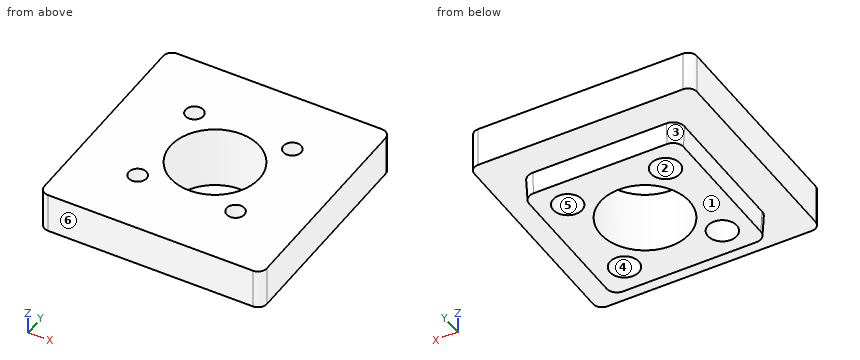
Autodesk Inventor part; units mm, degrees
ref_plane "YZ Plane" through (0, 0, 0) normal (1, 0, 0) x (0, 1, 0)
ref_plane "XZ Plane" through (0, 0, 0) normal (0, 1, 0) x (-1, 0, 0)
ref_plane "XY Plane" through (0, 0, 0) normal (0, 0, 1) x (1, 0, 0)
ref_plane "Arbeitsebene15" through (-38.58009, 58.540516, -23.010083) normal (0, 0, 1) x (1, 0, 0)
sketch "Skizze38" plane through (-38.58009, 58.540516, -23.010083) normal (0, 0, 1) x (1, 0, 0)
  circle A0 centre (27, 33.3) radius 3
  circle A1 centre (-8.3, 27) radius 3
  circle A2 centre (-2, -8.3) radius 3
  circle A3 centre (33.3, -2) radius 3
  circle A4 centre (27, -8.3) radius 3
  circle A5 centre (-8.3, -2) radius 3
  circle A6 centre (-2, 33.3) radius 3
  circle A7 centre (33.3, 27) radius 3
  line L0 (27.5, 29.5) -> (-2.5, 29.5)
  arc A8 (29.5, 27.5) -> (27.5, 29.5) centre (27.5, 27.5) ccw
  line L1 (29.5, 27.5) -> (29.5, -2.5)
  arc A9 (27.5, -4.5) -> (29.5, -2.5) centre (27.5, -2.5) ccw
  line L2 (-2.5, -4.5) -> (27.5, -4.5)
  arc A10 (-4.5, -2.5) -> (-2.5, -4.5) centre (-2.5, -2.5) ccw
  line L3 (-4.5, -2.5) -> (-4.5, 27.5)
  arc A11 (-2.5, 29.5) -> (-4.5, 27.5) centre (-2.5, 27.5) ccw
  circle A12 centre (33.5, 33.5) radius 2.5
  circle A13 centre (-8.5, -8.5) radius 2.5
  circle A14 centre (33.5, -8.5) radius 2.5
  circle A15 centre (-8.5, 33.5) radius 2.5
  line L4 (-11.75, -10.5) -> (-11.75, 8.25)
  arc A16 (-11.75, -10.5) -> (-10.5, -11.75) centre (-10.5, -10.5) ccw
  line L5 (8.25, -11.75) -> (-10.5, -11.75)
  line L6 (8.25, -13.877389) -> (8.25, -11.75)
  arc A17 (7.405556, -14.865216) -> (8.25, -13.877389) centre (7.25, -13.877389) ccw
  arc A18 (7.405556, -14.865216) -> (7.6, -17.35) centre (7.6, -16.1) ccw
  line L7 (17.4, -17.35) -> (7.6, -17.35)
  arc A19 (17.4, -17.35) -> (17.594444, -14.865216) centre (17.4, -16.1) ccw
  arc A20 (16.75, -13.877389) -> (17.594444, -14.865216) centre (17.75, -13.877389) ccw
  line L8 (16.75, -11.75) -> (16.75, -13.877389)
  line L9 (35.5, -11.75) -> (16.75, -11.75)
  arc A21 (35.5, -11.75) -> (36.75, -10.5) centre (35.5, -10.5) ccw
  line L10 (36.75, 6.487451) -> (36.75, -10.5)
  arc A22 (36.75, 6.487451) -> (36.55605, 6.521706) centre (36.65, 6.487451) ccw
  arc A23 (31.3, 7.45) -> (36.55605, 6.521706) centre (34.01, 7.45) ccw
  line L11 (31.3, 17.55) -> (31.3, 7.45)
  arc A24 (36.55605, 18.478294) -> (31.3, 17.55) centre (34.01, 17.55) ccw
  arc A25 (36.55605, 18.478294) -> (36.75, 18.512549) centre (36.65, 18.512549) ccw
  line L12 (36.75, 35.5) -> (36.75, 18.512549)
  arc A26 (36.75, 35.5) -> (35.5, 36.75) centre (35.5, 35.5) ccw
  line L13 (18.512549, 36.75) -> (35.5, 36.75)
  arc A27 (18.512549, 36.75) -> (18.478294, 36.55605) centre (18.512549, 36.65) ccw
  arc A28 (17.55, 31.3) -> (18.478294, 36.55605) centre (17.55, 34.01) ccw
  line L14 (7.45, 31.3) -> (17.55, 31.3)
  arc A29 (6.521706, 36.55605) -> (7.45, 31.3) centre (7.45, 34.01) ccw
  arc A30 (6.521706, 36.55605) -> (6.487451, 36.75) centre (6.487451, 36.65) ccw
  line L15 (-10.5, 36.75) -> (6.487451, 36.75)
  arc A31 (-10.5, 36.75) -> (-11.75, 35.5) centre (-10.5, 35.5) ccw
  line L16 (-11.75, 16.75) -> (-11.75, 35.5)
  line L17 (-13.877389, 16.75) -> (-11.75, 16.75)
  arc A32 (-14.865216, 17.594444) -> (-13.877389, 16.75) centre (-13.877389, 17.75) ccw
  arc A33 (-14.865216, 17.594444) -> (-17.35, 17.4) centre (-16.1, 17.4) ccw
  line L18 (-17.35, 7.6) -> (-17.35, 17.4)
  arc A34 (-17.35, 7.6) -> (-14.865216, 7.405556) centre (-16.1, 7.6) ccw
  arc A35 (-13.877389, 8.25) -> (-14.865216, 7.405556) centre (-13.877389, 7.25) ccw
  line L19 (-11.75, 8.25) -> (-13.877389, 8.25)
  line L20 (-2.5, 30.1) -> (27.5, 30.1)
  arc A36 (30.1, 27.5) -> (27.5, 30.1) centre (27.5, 27.5) ccw
  line L21 (30.1, 27.5) -> (30.1, -2.5)
  arc A37 (27.5, -5.1) -> (30.1, -2.5) centre (27.5, -2.5) ccw
  line L22 (27.5, -5.1) -> (-2.5, -5.1)
  arc A38 (-5.1, -2.5) -> (-2.5, -5.1) centre (-2.5, -2.5) ccw
  line L23 (-5.1, -2.5) -> (-5.1, 27.5)
  arc A39 (-2.5, 30.1) -> (-5.1, 27.5) centre (-2.5, 27.5) ccw
  point P0 (38.58009, -58.540516)
  dimension "d425" = 0.6
sketch "Skizze38 outline for Extrusion20" plane through (-38.58009, 58.540516, -23.010083) normal (0, 0, 1) x (1, 0, 0)
  arc A0 (-5.1, -2.5) -> (-2.5, -5.1) centre (-2.5, -2.5) ccw
  line L0 (-5.1, 27.5) -> (-5.1, -2.5)
  arc A1 (-2.5, 30.1) -> (-5.1, 27.5) centre (-2.5, 27.5) ccw
  line L1 (27.5, 30.1) -> (-2.5, 30.1)
  arc A2 (30.1, 27.5) -> (27.5, 30.1) centre (27.5, 27.5) ccw
  line L2 (30.1, -2.5) -> (30.1, 27.5)
  arc A3 (27.5, -5.1) -> (30.1, -2.5) centre (27.5, -2.5) ccw
  line L3 (-2.5, -5.1) -> (27.5, -5.1)
extrude "Extrusion20" add sketch "Skizze38 outline for Extrusion20" against normal blind 5 draft -3
sketch "Skizze39" plane through (-38.58009, 58.540516, -23.010083) normal (0, 0, 1) x (1, 0, 0)
  line L0 (-2.5, -5.1) -> (27.5, -5.1)
  arc A0 (27.5, -5.1) -> (30.1, -2.5) centre (27.5, -2.5) ccw
  line L1 (30.1, -2.5) -> (30.1, 27.5)
  arc A1 (30.1, 27.5) -> (27.5, 30.1) centre (27.5, 27.5) ccw
  line L2 (27.5, 30.1) -> (-2.5, 30.1)
  arc A2 (-2.5, 30.1) -> (-5.1, 27.5) centre (-2.5, 27.5) ccw
  line L3 (-5.1, 27.5) -> (-5.1, -2.5)
  arc A3 (-5.1, -2.5) -> (-2.5, -5.1) centre (-2.5, -2.5) ccw
  line L4 (17.5, -12.5) -> (35.5, -12.5)
  line L5 (-10.5, 37.5) -> (35.5, 37.5)
  line L6 (37.5, 35.5) -> (37.5, -10.5)
  line L7 (35.5, -12.5) -> (-10.5, -12.5)
  line L8 (-12.5, -10.5) -> (-12.5, 35.5)
  line L9 (-12.5, 37.5) -> (37.5, -12.5) construction
  line L10 (37.5, 37.5) -> (-12.5, -12.5) construction
  arc A4 (37.5, 35.5) -> (35.5, 37.5) centre (35.5, 35.5) ccw
  arc A5 (37.5, 35.5) -> (35.5, 37.5) centre (35.5, 35.5) ccw
  arc A6 (-10.5, 37.5) -> (-12.5, 35.5) centre (-10.5, 35.5) ccw
  arc A7 (-12.5, -10.5) -> (-10.5, -12.5) centre (-10.5, -10.5) ccw
  arc A8 (35.5, -12.5) -> (37.5, -10.5) centre (35.5, -10.5) ccw
  point P0 (38.58009, -58.540516)
  point P1 (12.5, 12.5)
  point P2 (35.5, -12.5)
  dimension "d428" = 50
  dimension "d429" = 50
  dimension "d430" = 2
extrude "Extrusion21" add sketch "Skizze39" along normal blind 9 contours A3 L3 A2 L2 A1 L1 A0 L0 | L7 A7 L8 A6 L5 A4 L6 A8 L4
sketch "Skizze40" plane through (-38.58009, 58.540516, -14.010083) normal (0, 0, 1) x (1, 0, 0)
  arc A0 (-10.5, 37.5) -> (-12.5, 35.5) centre (-10.5, 35.5) ccw
  line L0 (-12.5, 35.5) -> (-12.5, -10.5)
  arc A1 (-12.5, -10.5) -> (-10.5, -12.5) centre (-10.5, -10.5) ccw
  line L1 (-10.5, -12.5) -> (35.5, -12.5)
  arc A2 (35.5, -12.5) -> (37.5, -10.5) centre (35.5, -10.5) ccw
  line L2 (37.5, -10.5) -> (37.5, 35.5)
  arc A3 (37.5, 35.5) -> (35.5, 37.5) centre (35.5, 35.5) ccw
  line L3 (35.5, 37.5) -> (-10.5, 37.5)
  circle A4 centre (12.5, 12.5) radius 10
  line L4 (1.5, 23.5) -> (23.5, 23.5)
  line L5 (23.5, 23.5) -> (23.5, 1.5)
  line L6 (23.5, 1.5) -> (1.5, 1.5)
  line L7 (1.5, 1.5) -> (1.5, 23.5)
  line L8 (1.5, 23.5) -> (23.5, 1.5) construction
  line L9 (23.5, 23.5) -> (1.5, 1.5) construction
  circle A5 centre (1.5, 1.5) radius 1.6
  circle A6 centre (1.5, 23.5) radius 1.6
  circle A7 centre (23.5, 23.5) radius 1.6
  circle A8 centre (23.5, 1.5) radius 1.6
  dimension "d466" = 20
  dimension "d467" = 22
  dimension "d468" = 22
  dimension "d469" = 3.2
  dimension "d470" = 3.2
  dimension "d471" = 3.2
  dimension "d472" = 3.2
extrude "Extrusion22" cut sketch "Skizze40" against normal through all contours A4 | L7 A6 L4 | L4 A6 L7 | A7 L5 L4 | L4 L5 A7 | A5 L6 L7 | L7 L6 A5 | A8 L6 L5 | L5 L6 A8
sketch "Skizze43" plane through (-38.58009, 58.540516, -28.010083) normal (0, 0, -1) x (-1, 0, 0)
  circle A0 centre (-1.5, 23.5) radius 1.6
  circle A1 centre (-1.5, 1.5) radius 1.6
  circle A2 centre (-23.5, 23.5) radius 1.6
  circle A3 centre (-12.5, 12.5) radius 10
  circle A4 centre (-23.5, 1.5) radius 1.6
  line L0 (2.5, -4.837961) -> (-27.5, -4.837961)
  arc A5 (2.5, -4.837961) -> (4.837961, -2.5) centre (2.5, -2.5) ccw
  line L1 (4.837961, 27.5) -> (4.837961, -2.5)
  arc A6 (4.837961, 27.5) -> (2.5, 29.837961) centre (2.5, 27.5) ccw
  line L2 (-27.5, 29.837961) -> (2.5, 29.837961)
  arc A7 (-27.5, 29.837961) -> (-29.837961, 27.5) centre (-27.5, 27.5) ccw
  line L3 (-29.837961, -2.5) -> (-29.837961, 27.5)
  arc A8 (-29.837961, -2.5) -> (-27.5, -4.837961) centre (-27.5, -2.5) ccw
  circle A9 centre (-23.5, 1.5) radius 1.6
  circle A10 centre (-1.5, 23.5) radius 1.6
  circle A11 centre (-1.5, 1.5) radius 1.6
  point P0 (-38.58009, -58.540516)
  point P1 (-23.5, 1.5)
  point P2 (-23.5, 23.5)
  point P3 (-1.5, 23.5)
  point P4 (-1.5, 1.5)
hole "Bohrung11" at (-15.08009, 60.040516, -28.010083) at (-15.08009, 82.040516, -28.010083) at (-37.08009, 82.040516, -28.010083) at (-37.08009, 60.040516, -28.010083) direction (0, 0, 1) diameter 4 end through all counterbore diameter 6.5 counterbore depth 8
equation "\"d_i\" = 40"
equation "\"d_o\" = 40"
equation "\"d_part\" = 50"
equation "\"d6\" = 0"
equation "\"d7\" = 0"
equation "\"d8\" = 0"
equation "\"d9\" = 0"
equation "\"d13\" = 0"
equation "\"d14\" = 0"
equation "\"d20\" = 0"
equation "\"d21\" = 0"
equation "\"d22\" = 0"
equation "\"d23\" = 0"
equation "\"d24\" = 0"
equation "\"d25\" = 3"
equation "\"d26\" = 0"
equation "\"d27\" = 0"
equation "\"d28\" = 0"
equation "\"d29\" = 0"
equation "\"d30\" = 0"
equation "\"d31\" = 0"
equation "\"d32\" = 0"
equation "\"d33\" = 0"
equation "\"d34\" = 0"
equation "\"d46\" = 0"
equation "\"d47\" = 0"
equation "\"d48\" = 0"
equation "\"d50\" = 0"
equation "\"d51\" = 0"
equation "\"d52\" = 0"
equation "\"d53\" = 0"
equation "\"d54\" = 0"
equation "\"d55\" = 0"
equation "\"d56\" = 0"
equation "\"d57\" = 0"
equation "\"d58\" = 0"
equation "\"d59\" = 0"
equation "\"magnet_offset\" = 0"
equation "\"screw_offset\" = 0"
equation "\"mal_puzzle_offset\" = 0"
equation "\"fem_puzzle_offset\" = 0"
properties part number "20_Cube_Adapter_Zstage_motorized"
Read the model definition and answer for the solid it produces. Units are mm, in the model's axes. Face numbers are marked on the shaded views. A direction names the side the tool comes from. Round coordinates to 2 decimals unless told otherwise and drop trailing zeros. Write each loop counter-clockwise with the first axis right and the second up, starting at its lowest first coordinate (ties: lowest second). Pieces come first, ordered by that corner, then holes. Notation, with made-up numbers: (30.25, -27.5) -> (54.25, -27.5) arc R22 cw to (54.25, 2.5) -> close; hole circle Ø1 at (77.25, -36.75). An arc over 180 degrees is marked (long way). Answer in a Markdown table with one row per item. Add a question column.
1) Consider line 1 (X direction, y = 70.5, z = -17.5); line 2 (Y direction, x = -35, z = -26.5); line 3 (X direction, y = 58, z = -22). Determine where each line is inside the solid, lowest interval first.
2) Which of the six approach directions +Z, -Z, +X, -X, +Y, -Y give full straight-line access (tool end or side, diameter ignored) to the marked faces 1 and 2?
3) Find section A-A, the plane y = 73. Determine the outline of the cut face in (x, z), and give its area (3 significant figures).
4) Given P1, Ø3, axis at x = -38, y = 82, coming from the -Z side; P2, Ø1, axis at x = -32.5, z = -25.5, coming from the -Y side; P3, Ø3, axis at x = -37.08, y = 82.04, coming from the +Z side, each flat-ended and moving along its own axis, determine where each tip first touches the part or whether it passes through.
5) Find section B-B, the plane x = -24. Determine the outline of the cut face in (y, z).
6) Find section D-D, the plane z = -26. Determine the outline of the cut face in (x, y), and give its area (3 significant figures).
7) Find section C-C, the plane y = 83. Determine the outline of the cut face in (x, z), and give its area (3 significant figures).
8) Determine the mould class of the marked faces 3, 4, 5 and 6 for opening direction X: pulls with the +X half, pulls with the -X half, needs draft (parallel to the pull), parting line crosses it, or undercut.
Findings below:
| question | item | result |
|---|---|---|
| 1 | line 1 | -51.08 to -36.07, -16.09 to -1.08 |
| 1 | line 2 | 53.62 to 57.54, 62.54 to 66.52, 75.56 to 79.54, 84.54 to 88.46 |
| 1 | line 3 | -51.08 to -39.61, -34.55 to -17.61, -12.55 to -1.08 |
| 2 | face 1 | -Z, +X, -X, +Y, -Y |
| 2 | face 2 | -Z |
| 3 | outline | (-51.08, -23.01) -> (-43.68, -23.01) -> (-43.42, -28.01) -> (-35.89, -28.01) -> (-35.89, -14.01) -> (-51.08, -14.01) -> close; (-16.27, -28.01) -> (-8.74, -28.01) -> (-8.48, -23.01) -> (-1.08, -23.01) -> (-1.08, -14.01) -> (-16.27, -14.01) -> close |
| 3 | area | 350 mm² |
| 4 | P1 | z = -20.01 |
| 4 | P2 | y = 53.54 |
| 4 | P3 | through |
| 5 | outline | (46.04, -23.01) -> (53.44, -23.01) -> (53.7, -28.01) -> (61.26, -28.01) -> (61.26, -14.01) -> (46.04, -14.01) -> close; (80.82, -28.01) -> (88.38, -28.01) -> (88.64, -23.01) -> (96.04, -23.01) -> (96.04, -14.01) -> (80.82, -14.01) -> close |
| 6 | outline | (-43.52, 56.04) arc R2.44 ccw to (-41.08, 53.6) -> (-11.08, 53.6) arc R2.44 ccw to (-8.64, 56.04) -> (-8.64, 86.04) arc R2.44 ccw to (-11.08, 88.48) -> (-41.08, 88.48) arc R2.44 ccw to (-43.52, 86.04) -> close; hole circle Ø6.5 at (-37.08, 60.04); hole circle Ø6.5 at (-37.08, 82.04); hole circle Ø20 at (-26.08, 71.04); hole circle Ø6.5 at (-15.08, 60.04); hole circle Ø6.5 at (-15.08, 82.04) |
| 6 | area | 765 mm² |
| 7 | outline | (-51.08, -23.01) -> (-43.68, -23.01) -> (-43.42, -28.01) -> (-40.19, -28.01) -> (-40.19, -20.01) -> (-38.83, -20.01) -> (-38.83, -14.01) -> (-51.08, -14.01) -> close; (-35.33, -20.01) -> (-33.97, -20.01) -> (-33.97, -28.01) -> (-18.19, -28.01) -> (-18.19, -20.01) -> (-16.83, -20.01) -> (-16.83, -14.01) -> (-35.33, -14.01) -> close; (-13.33, -20.01) -> (-11.97, -20.01) -> (-11.97, -28.01) -> (-8.74, -28.01) -> (-8.48, -23.01) -> (-1.08, -23.01) -> (-1.08, -14.01) -> (-13.33, -14.01) -> close |
| 7 | area | 483 mm² |
| 8 | face 3 | pulls with the -X half |
| 8 | face 4 | undercut |
| 8 | face 5 | undercut |
| 8 | face 6 | needs draft |
